Autodesk Inventor part; units mm, degrees
ref_plane "YZ Plane" through (0, 0, 0) normal (1, 0, 0) x (0, 1, 0)
ref_plane "XZ Plane" through (0, 0, 0) normal (0, 1, 0) x (-1, 0, 0)
ref_plane "XY Plane" through (0, 0, 0) normal (0, 0, 1) x (1, 0, 0)
ref_plane "Work Plane1" through (-52.4749, 258.6532, -6.397) normal (0, 0, 1) x (0, -1, 0)
sketch "Sketch1" plane through (-52.4749, 258.6532, -6.397) normal (0, 0, 1) x (0, -1, 0)
  line L0 (0.0003, 0.0039) -> (-20.2411, 10.8651)
  arc A0 (-20.2411, 10.8651) -> (-35.6461, -2.9695) centre (-25.4455, 1.1661) ccw
  line L1 (-35.6461, -2.9695) -> (42.4229, -195.5278)
  line L2 (42.4229, -195.5278) -> (42.4229, -219.8278)
  line L3 (42.4229, -219.8278) -> (81.4481, -219.8278)
  line L4 (81.4481, -219.8278) -> (168.2058, -219.8263)
  line L5 (168.2058, -219.8263) -> (207.231, -219.8261)
  line L6 (207.231, -219.8261) -> (207.2309, -195.5273)
  ellipse E0 centre (186.2274, -195.5271) end of major axis (212.7883, -195.527) minor radius 0.0003 (207.231, -195.5268) -> (207.2309, -195.5273) ccw
  line L7 (207.231, -195.5268) -> (285.3, -2.9593)
  arc A1 (285.3, -2.9593) -> (269.9065, 10.8669) centre (275.106, 1.1734) ccw
  line L8 (269.9065, 10.8669) -> (249.6555, 0.0046)
  arc A2 (246.3474, -0.8266) -> (249.6555, 0.0046) centre (246.3474, 6.172) ccw
  line L9 (246.3474, -0.8266) -> (234.7987, -0.8277)
  arc A3 (234.7987, -0.8277) -> (224.1037, -11.8268) centre (235.1053, -11.8251) ccw
  line L10 (224.1037, -11.8268) -> (224.1037, -23.8268)
  line L11 (224.1037, -23.8268) -> (25.5516, -23.8268)
  line L12 (25.5516, -23.8268) -> (25.5516, -11.8268)
  arc A4 (25.5516, -11.8268) -> (14.3466, -0.8277) centre (14.5506, -11.8268) ccw
  line L13 (14.3466, -0.8277) -> (3.3091, -0.8277)
  arc A5 (0.0003, 0.0039) -> (3.3091, -0.8277) centre (3.3091, 6.1703) ccw
  circle A6 centre (275.1036, 1.1723) radius 4.5971
  circle A7 centre (235.1053, -11.8251) radius 4.1019
  circle A8 centre (14.5506, -11.8268) radius 4.101
  circle A9 centre (61.9506, -207.5286) radius 4.1026
  circle A10 centre (187.7028, -207.5216) radius 4.1055
  circle A11 centre (-25.4489, 1.1708) radius 4.0986
  circle A12 centre (-25.4489, 1.1708) radius 30
  point P0 (258.6534, 52.4739)
  dimension "d0" = 60
extrude "Extrusion1" add sketch "Sketch1" along normal blind 16 contours A5 L13 A12 L1 A0 L0 | L0 A0 L1 A12 L13 A5 | A11
chamfer "Chamfer1" distance 3 angle 45 2 edges at (-51.3043, 314.1021, -6.3967) (-51.3043, 314.102, 9.6033)
sketch "Sketch2" plane through (-51.3042, 284.102, 9.6032) normal (0, 0, 1) x (1, 0, 0)
  circle A0 centre (0, 0) radius 27
  circle A1 centre (-0.0044, 0.002) radius 4.0977
  circle A2 centre (-0.0044, 0.002) radius 11
  point P0 (51.3042, -284.102)
  dimension "d8" = 22
extrude "Extrusion2" cut sketch "Sketch2" against normal through all contours A1 | A2
properties part number "Wheel"
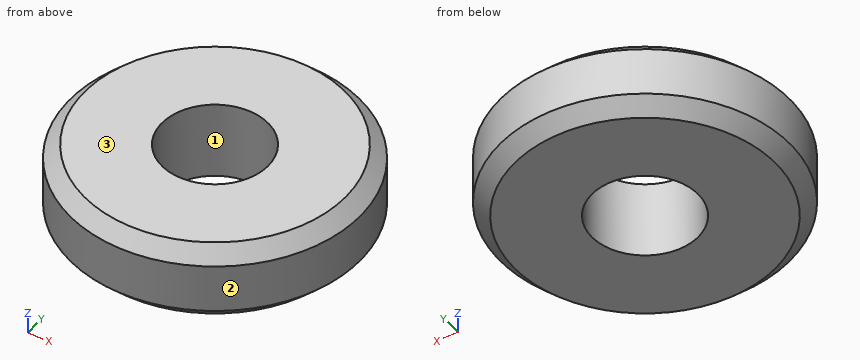
For this review, take the finished solid that the model builds, in its own axes (mm). Face numbers are marked on the shaded views. Round coordinates to 2 decimals unless told otherwise and drop trailing zeros. Order: outer loops, then holes, each group sorted by start corner. A loop starts at its lowest first (then second) coordinate and runs counter-clockwise, first axis right, second up.
Q1. Wall thickness on line 1 (Y direction, x = -60, z = -5); line 2 (Y direction, x = -42.5, z = -2.5); line 3 (X direction, y = 277, z = 4): over which ranges is each line inside the solid? List them lowest first.
Findings below:
line 1: y = 257.07 to 277.36, 290.85 to 311.13
line 2: y = 255.42 to 277.52, 290.69 to 312.78
line 3: x = -80.45 to -59.71, -42.91 to -22.16
Q2. We need section A-A, the plane z = 8.5. Give the boundary of the cut face in (x, y).
Findings below:
outline: circle Ø56.21 at (-51.3, 284.1); hole circle Ø22 at (-51.31, 284.1)
Q3. Insertion check: P1, Ø1, axis at y = 302.5, z = 2.5, coming from the +X side; P2, Ø1, axis at x = -65, z = -3.5, coming from the +Y side; P3, Ø2, axis at x = -46, z = 5.5, coming from the -Y side. Each pin has a flat end and moves straight along its axis. Give the tip position at first contact, or say it passes through.
Findings below:
P1: stops at x = -27.23
P2: stops at y = 311.04
P3: stops at y = 254.41
Q4. Mouldability with a two-part tool opening along Y and no side actions: class the marked faces 1, 2 and 3 as pulls with the +Y half, pulls with the -Y half, needs draft (parallel to the pull), parting line crosses it, or undercut.
Findings below:
face 1: undercut
face 2: parting line crosses it
face 3: needs draft
Q5. We need section B-B, the plane z = -5. Give the boundary of the cut face in (x, y), plus the area to 3 significant figures.
Findings below:
outline: circle Ø56.79 at (-51.3, 284.1); hole circle Ø22 at (-51.31, 284.1)
area: 2,150 mm2
